Read the model definition and answer for the solid it produces. Units are mm, in the model's axes. A direction names the side the tool comes from. Round coordinates to 2 decimals unless told otherwise and drop trailing zeros. Order: outer loops, then holes, each group sorted by start corner. A loop starts at its lowest first (then second) coordinate and runs counter-clockwise, first axis right, second up. Notation, with made-up numbers: (89.25, -21.5) -> (131.25, -21.5) arc R22 ccw to (131.25, -7.5) -> close; hole circle Ø4 at (81, -10.5). An arc over 180 degrees is marked (long way). Answer as a JSON object with one key per item and string values. Group by question number.
Item 1: Given P1, Ø1.6, axis at x = 53.5, z = -0.5, coming from the -Y side; P2, Ø1.6, axis at y = -23, z = 0, coming from the +X side; P3, Ø1, axis at y = -9.5, z = 0, coming from the -X side, each flat-ended and moving along its own axis, determine where each tip first touches the part or whether it passes through.
Item 2: For faces 1 (the flat face through (22.788, -23, 0)), 2 (the flat face through (49, -21.7, 0)), 3 (the flat face through (15.288, -23, 0)), 4 (the flat face through (29, -13.14, 0)), determine the directions among +Z, -Z, +X, -X, +Y, -Y from which every point of the face is accessible in a straight line to the end or side of a thin tool.
Item 3: Section D-D, the plane y = -17.5 is taken. Write down the section's boundary in (x, z), plus the area to 3 significant figures.
Item 4: Section C-C, the plane x = 18 is taken. Write down the section's boundary in (y, z), plus the area to 3 significant figures.
Item 5: Section B-B, the plane z = 0.6 is taken. Write down the section's boundary in (x, y).
Item 6: Section A-A, the plane y = -23.25 is taken. Write down the section's boundary in (x, z).
Item 7: Consider probe 1 along X at (y, z) = (-22.5, -0.3); probe 2 along Y at (x, z) = (51.5, -0.8); probe 3 along Y at (x, z) = (79, 1.55). Determine where each line is inside the solid, lowest interval first. Write a range as from..to.
Autodesk Inventor part; units mm, degrees
ref_plane "YZ Plane" through (0, 0, 0) normal (1, 0, 0) x (0, 1, 0)
ref_plane "XZ Plane" through (0, 0, 0) normal (0, 1, 0) x (-1, 0, 0)
ref_plane "XY Plane" through (0, 0, 0) normal (0, 0, 1) x (1, 0, 0)
sketch "Sketch1" plane through (0, 0, 0) normal (0, 0, 1) x (1, 0, 0)
  line L0 (58, -6.1405) -> (122, -6.1405)
  line L1 (122, -6.1405) -> (122, -10.6498)
  line L2 (122, -10.6498) -> (57.892, -21.6998)
  line L3 (4.088, -21.6998) -> (15.288, -21.6998)
  line L4 (15.288, -21.6998) -> (15.288, -24.8998)
  line L5 (15.288, -24.8998) -> (22.788, -24.8998)
  line L6 (22.788, -24.8998) -> (22.788, -21.6998)
  line L7 (32.788, -21.6998) -> (32.788, -24.8998)
  line L8 (40.288, -24.8998) -> (40.288, -21.6998)
  line L9 (58, -6.1405) -> (122, -6.1405)
  line L10 (122, -6.1405) -> (122, -10.6498)
  line L11 (57.892, -21.6998) -> (122, -10.6498)
  line L12 (57.892, -21.6998) -> (40.288, -21.6998)
  line L13 (40.288, -24.8998) -> (40.288, -21.6998)
  line L14 (40.288, -24.8998) -> (32.788, -24.8998)
  line L15 (32.788, -24.8998) -> (32.788, -21.6998)
  line L16 (32.788, -21.6998) -> (22.788, -21.6998)
  line L17 (22.788, -24.8998) -> (22.788, -21.6998)
  line L18 (15.288, -24.8998) -> (22.788, -24.8998)
  line L19 (15.288, -24.8998) -> (15.288, -21.6998)
  line L20 (15.288, -21.6998) -> (4.088, -21.6998)
  line L21 (58, -6.1405) -> (58, -13.1405)
  line L22 (4.088, -21.6998) -> (4.088, -13.1405)
  line L23 (4.088, -13.1405) -> (58, -13.1405)
  point P0 (0, 0)
  point P1 (0, 0)
  dimension "d1" = 11.2
  dimension "d2" = 7.5
  dimension "d3" = 10
  dimension "d4" = 7.5
  dimension "d15" = 21.6998
  dimension "d20" = 7
  dimension "d21" = 58
  dimension "d22" = 122
  dimension "d25" = 17.604
  dimension "d27" = 4.088
extrude "Plate1" add sketch "Sketch1" along normal mid plane 3.2
fillet "Corner Round3" radius 6 1 edges at (58, -13.1405, 0)
fillet "Corner Round4" radius 2 3 edges at (122, -6.1405, 0) (122, -10.6498, 0) (4.088, -13.1405, 0)
equation "\"d4\" = d2"
equation "\"d0\" = Thickness"
equation "\"BendRadius\" = Thickness"
equation "\"BendReliefWidth\" = Thickness"
equation "\"BendReliefDepth\" = 0.5 * Thickness"
equation "\"CornerReliefSize\" = 4 * Thickness"
equation "\"MinimumRemnant\" = 2 * Thickness"
equation "\"TransitionRadius\" = BendRadius"
equation "\"JacobiRadiusSize\" = BendRadius"
equation "\"GapSize\" = Thickness"
properties part number "SP9V1 Columna Freno" material "Stainless Steel"
Values found:
{
 "1": {"P1": "y = -21.7", "P2": "x = 40.29", "P3": "x = 57.27"},
 "2": {"face 1": "+Z, -Z, -Y", "face 2": "+Z, -Z, +X, -Y", "face 3": "+Z, -Z, -X, -Y", "face 4": "+Z, -Z, -X, +Y"},
 "3": {"outline": "(4.09, -1.6) -> (82.26, -1.6) -> (82.26, 1.6) -> (4.09, 1.6) -> close", "area": "250 mm2"},
 "4": {"outline": "(-24.9, -1.6) -> (-13.14, -1.6) -> (-13.14, 1.6) -> (-24.9, 1.6) -> close", "area": "37.6 mm2"},
 "5": {"outline": "(4.09, -21.7) -> (15.29, -21.7) -> (15.29, -24.9) -> (22.79, -24.9) -> (22.79, -21.7) -> (32.79, -21.7) -> (32.79, -24.9) -> (40.29, -24.9) -> (40.29, -21.7) -> (57.89, -21.7) -> (120.34, -10.94) arc R2 ccw to (122, -8.97) -> (122, -8.14) arc R2 ccw to (120, -6.14) -> (58, -6.14) -> (58, -7.14) arc R6 cw to (52, -13.14) -> (6.09, -13.14) arc R2 ccw to (4.09, -15.14) -> close"},
 "6": {"outline": "(15.29, -1.6) -> (22.79, -1.6) -> (22.79, 1.6) -> (15.29, 1.6) -> close; (32.79, -1.6) -> (40.29, -1.6) -> (40.29, 1.6) -> (32.79, 1.6) -> close"},
 "7": {"probe 1": "15.29..22.79, 32.79..40.29", "probe 2": "-21.7..-13.14", "probe 3": "-18.06..-6.14"}
}
